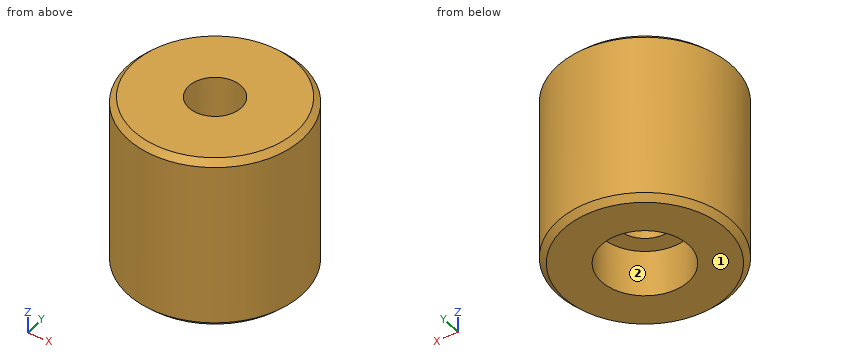
```python
from build123d import *

# Parameters (mm, degrees)
SKETCH_1_W                   = 30
SKETCH_1_H                   = 15
HOLE_WIZARD_M8_1_D           = 9
HOLE_WIZARD_M8_1_CBORE_D     = 15
HOLE_WIZARD_M8_1_CBORE_DEPTH = 8
CHAMFER_1_SIZE               = 1


with BuildPart() as part:
    # 草圖1 → 旋轉1 (revolve)
    with BuildSketch(Plane(origin=(0, 0, 0), x_dir=(0, 0, -1), z_dir=(1, 0, 0)), mode=Mode.PRIVATE) as revolve_1_sk:
        with Locations((15, 7.5)):
            Rectangle(SKETCH_1_W, SKETCH_1_H)
    revolve(revolve_1_sk.sketch.rotate(Axis((0, 0, 2.831513271), (0, 0, -1)), 90), axis=Axis((0, 0, 2.831513271), (0, 0, -1)))

    # M8 六角承窩頭蓋螺釘的柱孔1 (through all)
    with Locations(Plane(origin=(0, 0, -30), x_dir=(-1, 0, 0), z_dir=(0, 0, -1))):
        with Locations((0, 0)):
            CounterBoreHole(HOLE_WIZARD_M8_1_D / 2, HOLE_WIZARD_M8_1_CBORE_D / 2, HOLE_WIZARD_M8_1_CBORE_DEPTH)

    # 導角1
    chamfer_1_edges = [part.edges().sort_by_distance(p)[0] for p in [
        (-15, 0, -30),
        (-15, 0, 0),
    ]]
    chamfer(chamfer_1_edges, length=CHAMFER_1_SIZE)


solid = part.part
```
The listing builds one solid part. Answer for the finished solid, in the listing's coordinates (mm). Face numbers are marked on the shaded views. A direction names the side the tool comes from. Coordinates: 2 decimals unless noted, no trailing zeros. Write each loop counter-clockwise with the first axis right and the second up, starting at its lowest first coordinate (ties: lowest second). Pieces come first, ordered by that corner, then holes. Notation, with made-up numbers: M 12,9 L 54,9 A22 ccw 54,36 Z; hole C -37.5,62.5 d4. An arc over 180 degrees is marked long. Use a Markdown table: item, result. Add a question column.
1. Straight lines are drawn through the part: line 1 along Y through (x, z) = (0, -27.75); line 2 along Y through (x, z) = (0, -8); line 3 along X through (y, z) = (-3.5, -27.5). For each, find the intervals that lie inside material, in ascending order. Write a range as [from, to].
2. Which of the six approach directions +Z, -Z, +X, -X, +Y, -Y give full straight-line access (tool end or side, diameter ignored) to the marked faces 1 and 2?
3. Given P1, Ø2, axis at x = 11, z = -19, coming from the -Y side; P2, Ø7.5, axis at x = -3, y = -2, coming from the -Z side; P3, Ø10, axis at y = 8, z = -24.5, coming from the +X side, each flat-ended and moving along its own axis, determine where each tip first touches the part or whether it passes through.
4. Section C-C (z = -4.25) is taken. Give the vertices of the cut face in (x, y).
5. Section A-A (x = 0) is taken. Give the vertices of the cut face in (y, z), plus the area to 3 significant figures.
6. Section D-D (z = -24.5) is taken. Give the vertices of the cut face in (x, y).
Data:
| question | item | result |
|---|---|---|
| 1 | line 1 | y = [-15, -7.5], [7.5, 15] |
| 1 | line 2 | y = [-15, -4.5], [4.5, 15] |
| 1 | line 3 | x = [-14.59, -6.63], [6.63, 14.59] |
| 2 | face 1 | -Z, +X, -X, +Y, -Y |
| 2 | face 2 | -Z |
| 3 | P1 | stops at y = -11.18 |
| 3 | P2 | stops at z = -22 |
| 3 | P3 | stops at x = 14.7 |
| 4 | outline | C 0,0 d30; hole C 0,0 d9 |
| 5 | outline | M -15,-29 L -14,-30 L -7.5,-30 L -7.5,-22 L -4.5,-22 L -4.5,0 L -14,0 L -15,-1 Z; M 4.5,-22 L 7.5,-22 L 7.5,-30 L 14,-30 L 15,-29 L 15,-1 L 14,0 L 4.5,0 Z |
| 5 | area | 580 mm2 |
| 6 | outline | C 0,0 d30; hole C 0,0 d15 |
